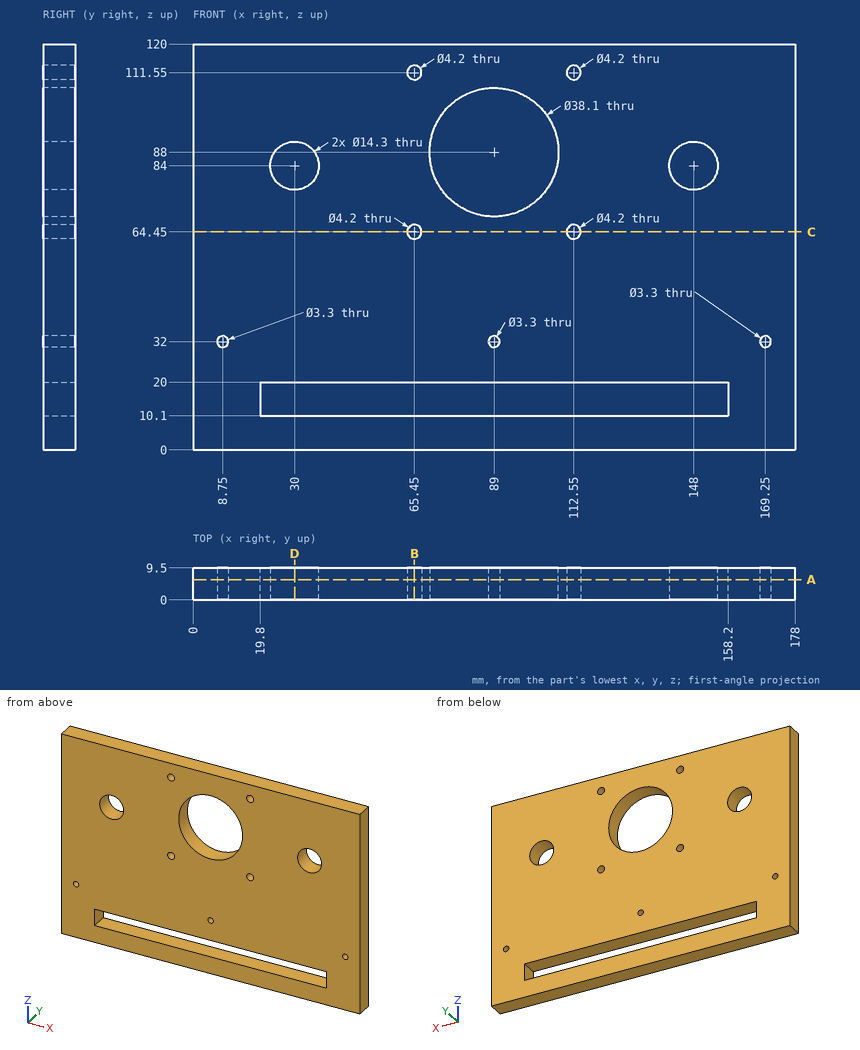
Here's the drawing with two shaded views (mm, measured from the low corner). I have some questions. Coordinates: 2 decimals unless noted, no trailing zeros. Order: outer loops, then holes, each group sorted by start corner. A loop starts at its lowest first (then second) coordinate and runs counter-clockwise, first axis right, second up.
Item 1: If we section it at A-A, the plane y = 6: Give the number of separate pieces and of enclosed holes in the cut face, then the cut area to 3 significant figures.
Response values:
separate pieces: 1
enclosed holes: 11
area: 18,400 mm2
Item 2: I need wall thicknesses on probe 1 along Z at (x, y) = (89, 2); probe 2 along Z at (x, y) = (148, 5); probe 3 along X at (y, z) = (5.75, 64.45). Which ranges of each line are inside material? Lowest first, please.
Response values:
probe 1: z = 0 to 10.1, 20 to 30.35, 33.65 to 68.95, 107.05 to 120
probe 2: z = 0 to 10.1, 20 to 76.85, 91.15 to 120
probe 3: x = 0 to 63.35, 67.55 to 110.45, 114.65 to 178
Item 3: If we section it at B-B, the plane x = 65.45: List the corners of the cut face in (y, z) for me.
Response values:
outline: (0, 0) - (9.5, 0) - (9.5, 10.1) - (0, 10.1) - close; (0, 20) - (9.5, 20) - (9.5, 62.35) - (0, 62.35) - close; (0, 66.55) - (9.5, 66.55) - (9.5, 109.45) - (0, 109.45) - close; (0, 113.65) - (9.5, 113.65) - (9.5, 120) - (0, 120) - close
Item 4: If we section it at D-D, the plane x = 30: List the corners of the cut face in (y, z) for me.
Response values:
outline: (0, 0) - (9.5, 0) - (9.5, 10.1) - (0, 10.1) - close; (0, 20) - (9.5, 20) - (9.5, 76.85) - (0, 76.85) - close; (0, 91.15) - (9.5, 91.15) - (9.5, 120) - (0, 120) - close
Item 5: If we section it at C-C, the plane z = 64.45: List the corners of the cut face in (x, y) for me, then the cut area to 3 significant figures.
Response values:
outline: (0, 0) - (63.35, 0) - (63.35, 9.5) - (0, 9.5) - close; (67.55, 0) - (110.45, 0) - (110.45, 9.5) - (67.55, 9.5) - close; (114.65, 0) - (178, 0) - (178, 9.5) - (114.65, 9.5) - close
area: 1,610 mm2
